Autodesk Inventor part; units mm, degrees
ref_plane "YZ Plane" through (0, 0, 0) normal (1, 0, 0) x (0, 1, 0)
ref_plane "XZ Plane" through (0, 0, 0) normal (0, 1, 0) x (-1, 0, 0)
ref_plane "XY Plane" through (0, 0, 0) normal (0, 0, 1) x (1, 0, 0)
sketch "Sketch1" plane through (0, 0, 0) normal (0, 1, 0) x (-1, 0, 0)
  circle A0 centre (0, 0) radius 2.6
  circle A1 centre (0, 0) radius 4.2
  line L0 (1.5, -3.923) -> (-1.5, -3.923)
  line L1 (-1.5, -3.923) -> (-1.5, -7.423)
  line L2 (-1.5, -7.423) -> (1.5, -7.423)
  line L3 (1.5, -7.423) -> (1.5, -3.923)
  line L4 (0, 0) -> (0, -7.423)
  arc A2 (2.9348, -3.0045) -> (1.5, -7.423) centre (6.4286, -6.5812) ccw
  arc A3 (-1.5, -7.423) -> (-2.9348, -3.0045) centre (-6.4286, -6.5812) ccw
  point P0 (1.5, -7.423)
  point P1 (-1.5, -5.7395)
  dimension "d0" = 5.2
  dimension "d1" = 1.6
  dimension "d2" = 1.5
  dimension "d3" = 3.5
  dimension "d4" = 5
  dimension "d6" = 5
extrude "Extrusion1" add sketch "Sketch1" along normal blind 3 contours A1 L0 | A1 L1 A3 | A2 L3 A1 | L0 L4 A1 | A1 L4 L2 A3 L1 | L3 A2 L2 L4 A1 | A1 L4 L0
fillet "Fillet2" radius 0.5 2 edges at (1.5, 1.5, -7.423) (-1.5, 1.5, -7.423)
chamfer "Chamfer1" distance 0.6 angle 45 1 edges at (2.6, 3, 0)
equation "\"d0\" = d"
equation "\"d6\" = d4"
equation "\"d7\" = dep"
equation "\"d\" = 5.2"
equation "\"dep\" = 3"
properties part number "thumbscrew_converter_M3"
CAD build for the part. Positions are in the model's coordinates, mm. Coordinates: 2 decimals unless noted, no trailing zeros. Loops run counter-clockwise (first coordinate to the right, second up) from the corner with the lowest first, then second, coordinate; pieces in that order, holes last. Notation, with made-up numbers: (-1.75, 29) - (13.25, 29) arc R7 cw to (13.25, 39) - close; hole circle Ø4 at (55.25, 20). An arc over 180 degrees is marked (long way). Use CSV: the item, a comma, the result in double quotes. Start each with the question number.
Q1. Two-plate mould, pull along X, no slides. Class faces 1 (the cylindrical face through (-1.752, 1.479, -4.813)), 2 (the flat face through (0, 1, -7.423)), 3 (the cylindrical face through (0.338, 1.183, -2.578)), 4 (the cylindrical face through (0.1, 1.5, 4.2)): +X half, -X half, draft (parallel to the pull), parting line (faces both ways), or undercut.
Q2. Cut at A-A, the plane z = 0. List the corners of the cut face in (x, y).
Q3. Drop a flat-ended pin along its axis: P1, Ø1.5, axis at y = 2, z = -2.5, coming from the -X side. Give the stop position or say it passes through.
Q4. Cut at B-B, the plane x = 0. List the corners of the cut face in (y, z), then the cut area to 3 significant figures.
Q5. Cut at D-D, the plane z = -5.5. List the corners of the cut face in (x, y).
Q6. Probe probe 1 along Z at (x, y) = (0, 1.65); probe 2 along X at (y, z) = (0.65, 0); probe 3 along X at (y, z) = (0.8, -6.25). List the from-to ranges inside material, lowest first. Write a range as from..to.
Q7. Cut at C-C, the plane y = 2.1. List the corners of the cut face in (x, z).
Here are the results:
1,face 1,"-X half"
1,face 2,"draft"
1,face 3,"undercut"
1,face 4,"parting line"
2,outline,"(-4.2, 0) - (-2.6, 0) - (-2.6, 2.4) - (-3.2, 3) - (-4.2, 3) - close; (2.6, 0) - (4.2, 0) - (4.2, 3) - (3.2, 3) - (2.6, 2.4) - close"
3,P1,"x = -3.82"
4,outline,"(0, -7.42) - (3, -7.42) - (3, -3.2) - (2.4, -2.6) - (0, -2.6) - close; (0, 2.6) - (2.4, 2.6) - (3, 3.2) - (3, 4.2) - (0, 4.2) - close"
4,area,"18.9 mm2"
5,outline,"(-1.55, 0) - (1.55, 0) - (1.55, 3) - (-1.55, 3) - close"
6,probe 1,"-7.42..-2.6, 2.6..4.2"
6,probe 2,"-4.2..-2.6, 2.6..4.2"
6,probe 3,"-1.44..1.44"
7,outline,"(-2.93, -3) arc R5 cw to (-1.44, -6.89) arc R0.5 ccw to (-0.94, -7.42) - (0.94, -7.42) arc R0.5 ccw to (1.44, -6.89) arc R5 cw to (2.93, -3) arc R4.2 ccw (long way) to start; hole circle Ø5.2 at (0, 0)"
